Design review of the part built by this model. Coordinates are the model's own, in mm. Give positions to 0.01 mm unless a question says otherwise; leave off trailing zeros. Order: outer loops, then holes, each group sorted by start corner. A loop starts at its lowest first (then second) coordinate and runs counter-clockwise, first axis right, second up. Notation, with made-up numbers: M -29,26 L -15,26 A18 cw -15,37 Z; hole C -8,83 d1. An arc over 180 degrees is marked long. Answer as a JSON object with one key per item and string values.
from build123d import *

# Parameters (mm, degrees)
SKETCH1_R           = 4.762500002
SKETCH1_W           = 38.8
SKETCH1_H           = 40.878125
SKETCH1_R_2         = 3.175
BOSS_EXTRUDE1_DEPTH = 6.35
FILLET1_R           = 6.35


with BuildPart() as part:
    # Sketch1 → Boss-Extrude1 (new body)
    with BuildSketch(Plane(origin=(0, 0, 0), x_dir=(0, 0, -1), z_dir=(1, 0, 0))):
        Polygon((19.4, 20.4390625), (-19.4, 20.4390625), (-19.4, 77.846455089), (-19.4, 116.646455089), (19.4, 116.646455089), (19.4, 77.846455095), align=None)
        with Locations((0, 97.246455089)):
            Circle(SKETCH1_R, mode=Mode.SUBTRACT)
        Rectangle(SKETCH1_W, SKETCH1_H)
        with Locations((13.05, -13.748956991)):
            Circle(SKETCH1_R_2, mode=Mode.SUBTRACT)
        with Locations((-13.05, -13.748956991)):
            Circle(SKETCH1_R_2, mode=Mode.SUBTRACT)
        with Locations((13.05, 13.748956991)):
            Circle(SKETCH1_R_2, mode=Mode.SUBTRACT)
        with Locations((-13.05, 13.748956991)):
            Circle(SKETCH1_R_2, mode=Mode.SUBTRACT)
    extrude(amount=BOSS_EXTRUDE1_DEPTH)

    # Fillet1
    fillet1_edges = [part.edges().sort_by_distance(p)[0] for p in [
        (3.175, 116.646455089, 19.4),
        (3.175, 116.646455089, -19.4),
    ]]
    fillet(fillet1_edges, radius=FILLET1_R)


solid = part.part
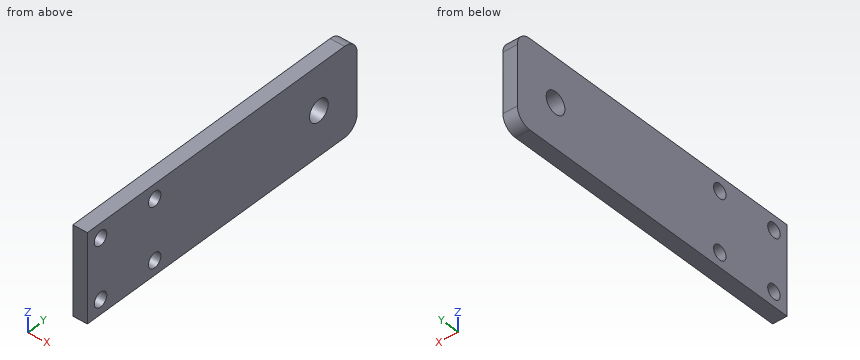
(1) We need section B-B (x = 5). Count the separate pieces of the cut face and the enclosed holes in it, plus the area to 3 significant figures.
Checked values:
{"separate pieces": "1", "enclosed holes": "5", "area": "5,100 mm^2"}
(2) To check wall thickness, follow L1, parallel to Y at x = 3.25, z = 13.05; L2, parallel to Z at x = 2.75, y = 14.5; L3, parallel to Z at x = 3, y = 15.5. State the ranges of each line that lie inside material, in increasing order. Write a range as from..to.
Checked values:
{"L1": "y = -20.44..-16.92, -10.57..10.57, 16.92..116.65", "L2": "z = -19.4..-16.13, -9.97..9.97, 16.13..19.4", "L3": "z = -19.4..-15.7, -10.4..10.4, 15.7..19.4"}
(3) We need section A-A (z = 0). Write out the cut boundary in (x, y).
Checked values:
{"outline": "M 0,-20.44 L 6.35,-20.44 L 6.35,92.48 L 0,92.48 Z; M 0,102.01 L 6.35,102.01 L 6.35,116.65 L 0,116.65 Z"}
